CAD build for the part. Positions are in the model's coordinates, mm. A direction names the side the tool comes from. Round coordinates to 2 decimals unless told otherwise and drop trailing zeros. Loops run counter-clockwise (first coordinate to the right, second up) from the corner with the lowest first, then second, coordinate; pieces in that order, holes last. Notation, with made-up numbers: M 30.25,14.5 L 44.25,14.5 A11 cw 44.25,27.5 Z; hole C 65.25,75.25 d4. An arc over 180 degrees is marked long. Use a Markdown table: item, result. Add a question column.
(1) Flat gauge pins, fed straight in: P1, Ø1.5, axis at x = -16.5, y = 3.5, coming from the -Z side; P2, Ø2, axis at x = -26.5, y = 4.5, coming from the +Z side; P3, Ø0.9, axis at y = 5, z = 2, coming from the -X side. Where does each tip first touch, or does it go through?
(2) Wall check: L1, parallel to Z at x = 0, y = 3.1; L2, parallel to X at y = 4.2, z = 11; L3, parallel to Y at x = -53.5, z = 24. Give the ranges that are in metal, low to high.
(3) Which spindle directions (+Z, -Z, +X, -X, +Y, -Y) get a long thin tool onto all of the face, cutting with end or side? Do faces 1 (the face through (-50, 4, 4)), 2 (the face through (-50.544, 3.493, 7.584)), 3 (the face through (12.236, 3, 4)), 4 (the face through (-18, 4, 11.537)). Say none if no direction does.
(4) Band-saw the part on D-D, the plane x = 0.5. Write the cut outline in (y, z), and give its area (3 significant figures).
(5) Band-saw the part on A-A, the plane x = -44.5. Write the cut outline in (y, z), and give its area (3 significant figures).
(6) Band-saw the part on B-B, the plane z = 13.5. Write the cut outline in (x, y).
(7) Two-plate mould, pull along X, no slides. Class faces 5 (the face through (11.785, 5.572, 3.827)), 6 (the face through (-57.764, 1, 4)), 7 (the face through (20.474, 1.639, 28.092)): released by +X, released by -X, zero draft, split by the parting line, or undercut.
(8) Band-saw the part on C-C, the plane z = -2.5. Write the cut outline in (x, y), and give its area (3 significant figures).
from build123d import *

# Parameters (mm, degrees)
SKETCH1_W               = 80
SKETCH1_H               = 50
BOSS_EXTRUDE1_DEPTH     = 2
SKETCH2_W               = 60
SKETCH2_H               = 30
SKETCH2_W_2             = 50
SKETCH2_H_2             = 15
BOSS_EXTRUDE4_DEPTH     = 4
SKETCH3_W               = 50
SKETCH3_H               = 15
BOSS_EXTRUDE5_DEPTH     = 1
BOSS_EXTRUDE6_DEPTH     = 1
FILLET2_R               = 1
FILLET3_R               = 1.5
ADVANCEDHOLE1_START     = 1.2888
ADVANCEDHOLE1_OUTLINE_R = 1.5875
ADVANCEDHOLE1_DEPTH     = 0.7112


# Read off the part's stored shape, not the designer's step: AdvancedHole1
with BuildPart() as part:
    # Sketch1 → Boss-Extrude1 (new body)
    with BuildSketch(Plane(origin=(0, 0, 0), x_dir=(1, 0, 0), z_dir=(0, 1, 0))):
        with Locations((-17.763975155, -4.037267081)):
            Rectangle(SKETCH1_W, SKETCH1_H)
    extrude(amount=BOSS_EXTRUDE1_DEPTH)

    # Sketch2 → Boss-Extrude4 (add)
    with BuildSketch(Plane(origin=(0, 2, 0), x_dir=(1, 0, 0), z_dir=(0, 1, 0))):
        with Locations((-17.763975155, -4.037267081)):
            Rectangle(SKETCH2_W, SKETCH2_H)
        with Locations((-17.763975155, -4.037267081)):
            Rectangle(SKETCH2_W_2, SKETCH2_H_2, mode=Mode.SUBTRACT)
    extrude(amount=BOSS_EXTRUDE4_DEPTH)

    # Sketch3 → Boss-Extrude5 (add)
    with BuildSketch(Plane(origin=(0, 2, 0), x_dir=(1, 0, 0), z_dir=(0, 1, 0))):
        with Locations((-17.763975155, -4.037267081)):
            Rectangle(SKETCH3_W, SKETCH3_H)
    extrude(amount=BOSS_EXTRUDE5_DEPTH)

    # Sketch4 → Boss-Extrude6 (add)
    with BuildSketch(Plane(origin=(0, 3, 0), x_dir=(1, 0, 0), z_dir=(0, 1, 0))):
        Polygon((-47.763975155, 0.962732919), (-47.763975155, -9.037267081), (-53.40213088, -6.089387941), (-53.40213088, -1.089387941), align=None)
    extrude(amount=BOSS_EXTRUDE6_DEPTH)

    # Fillet2
    fillet2_edges = [part.edges().sort_by_distance(p)[0] for p in [
        (-17.763975155, 6, 11.537267081),
        (-17.763975155, 6, -3.462732919),
    ]]
    fillet(fillet2_edges, radius=FILLET2_R)

    # Fillet3
    fillet3_edges = [part.edges().sort_by_distance(p)[0] for p in [
        (-47.763975155, 6, 4.037267081),
        (-17.763975155, 6, 19.037267081),
        (12.236024845, 6, 4.037267081),
        (-17.763975155, 6, -10.962732919),
    ]]
    fillet(fillet3_edges, radius=FILLET3_R)

    # AdvancedHole1 outline → AdvancedHole1 (cut)
    with BuildSketch(Plane(origin=(0, 0, 0), x_dir=(1, 0, 0), z_dir=(0, 1, 0)).offset(ADVANCEDHOLE1_START)):
        with Locations((19.741560812, -26.683343296)):
            Circle(ADVANCEDHOLE1_OUTLINE_R)
        with Locations((-55.139734181, -26.683343296)):
            Circle(ADVANCEDHOLE1_OUTLINE_R)
        with Locations((19.741560812, 18.219478311)):
            Circle(ADVANCEDHOLE1_OUTLINE_R)
        with Locations((-55.139734181, 18.219478311)):
            Circle(ADVANCEDHOLE1_OUTLINE_R)
    extrude(amount=ADVANCEDHOLE1_DEPTH, mode=Mode.SUBTRACT)


solid = part.part
Return value:
| question | item | result |
|---|---|---|
| 1 | P1 | z = -10.96 |
| 1 | P2 | z = 19.04 |
| 1 | P3 | x = -47.76 |
| 2 | L1 | -10.96 to -3.46, 11.54 to 19.04 |
| 2 | L2 | -47.76 to -42.76, 7.24 to 12.24 |
| 2 | L3 | 0 to 2 |
| 3 | face 1 | +Z, -Z, -X, +Y |
| 3 | face 2 | +Z, -X, +Y |
| 3 | face 3 | +Z, -Z, +X, +Y |
| 3 | face 4 | +Y |
| 4 | outline | M 0,-20.96 L 2,-20.96 L 2,-10.96 L 4.5,-10.96 A1.5 ccw 6,-9.46 L 6,-4.46 A1 ccw 5,-3.46 L 3,-3.46 L 3,11.54 L 5,11.54 A1 ccw 6,12.54 L 6,17.54 A1.5 ccw 4.5,19.04 L 2,19.04 L 2,29.04 L 0,29.04 Z |
| 4 | area | 174 mm^2 |
| 5 | outline | M 0,-20.96 L 2,-20.96 L 2,-10.96 L 4.5,-10.96 A1.5 ccw 6,-9.46 L 6,17.54 A1.5 ccw 4.5,19.04 L 2,19.04 L 2,29.04 L 0,29.04 Z |
| 5 | area | 219 mm^2 |
| 6 | outline | M -57.76,0 L 22.24,0 L 22.24,2 L 12.24,2 L 12.24,4.5 A1.5 ccw 10.74,6 L -46.26,6 A1.5 ccw -47.76,4.5 L -47.76,2 L -57.76,2 Z |
| 7 | face 5 | released by +X |
| 7 | face 6 | released by -X |
| 7 | face 7 | undercut |
| 8 | outline | M -57.76,0 L 22.24,0 L 22.24,2 L 12.24,2 L 12.24,4.5 A1.5 ccw 10.74,6 L 7.24,6 L 7.24,3 L -42.76,3 L -42.76,6 L -46.26,6 A1.5 ccw -47.76,4.5 L -47.76,2 L -57.76,2 Z |
| 8 | area | 249 mm^2 |
